from build123d import *

# Parameters (mm, degrees)
F1_DEPTH = 25.4
F2_W     = 101.6
F2_H     = 25.4
F3_DEPTH = 50.8
F4_W     = 25.4
F4_H     = 25.4
F5_DEPTH = 25.401


with BuildPart() as f1:
    # F0 (on Top) → F1 (new body)
    with BuildSketch(Plane.XY):
        with BuildLine():
            ThreePointArc((-50.8, -38.1), (0, -88.9), (50.8, -38.1))
            Line((50.8, -38.1), (25.4, -38.1))
            ThreePointArc((25.4, -38.1), (0, -63.5), (-25.4, -38.1))
            Line((-25.4, -38.1), (-50.8, -38.1))
        make_face()
        with BuildLine():
            ThreePointArc((-50.8, -38.1), (0, 12.7), (50.8, -38.1))
            Line((50.8, -38.1), (50.8, 38.1))
            Line((50.8, 38.1), (-50.8, 38.1))
            Line((-50.8, 38.1), (-50.8, -38.1))
        make_face()
        with BuildLine():
            Line((25.4, -38.1), (50.8, -38.1))
            ThreePointArc((50.8, -38.1), (0, 12.7), (-50.8, -38.1))
            Line((-50.8, -38.1), (-25.4, -38.1))
            ThreePointArc((-25.4, -38.1), (0, -12.7), (25.4, -38.1))
        make_face()
    extrude(amount=F1_DEPTH)

    # F2 (on face) → F3 (join)
    with BuildSketch(Plane.XY.offset(25.4)):
        with Locations((0, 25.4)):
            Rectangle(F2_W, F2_H)
    extrude(amount=F3_DEPTH)

    # F4 (on face) → F5 (cut, through all)
    with BuildSketch(Plane.XZ.offset(-12.7)):
        with Locations((-38.1, 63.5)):
            Rectangle(F4_W, F4_H)
    extrude(amount=-F5_DEPTH, mode=Mode.SUBTRACT)


solid = f1.part
CAD build for the part. Positions are in the model's coordinates, mm. A direction names the side the tool comes from. Round coordinates to 2 decimals unless told otherwise and drop trailing zeros. Order: outer loops, then holes, each group sorted by start corner. A loop starts at its lowest first (then second) coordinate and runs counter-clockwise, first axis right, second up. Notation, with made-up numbers: (-39, 48) -> (-13, 48) arc R16 cw to (-13, 61) -> close; hole circle Ø9 at (61, 41.25). An arc over 180 degrees is marked (long way). Write item = value, one per line. Start each with the question number.
(1) Probe line 1 (Y direction, x = 0, z = 19.5); line 2 (Y direction, x = -43, z = 32.5); line 3 (Z direction, x = -5, y = 12.5). List the from-to ranges inside material, lowest first. Write a range as [from, to].
(2) Pull direction X, two halves, no side cores. Call faces 4 (the cylindrical face through (3.307, -12.916, 12.522)), 5 (the flat face through (-1, 12.7, 50)), 6 (the flat face through (50.8, 16, 29)), 7 (the flat face through (-25.4, 25, 63)): released by +X, released by -X, zero draft, split by the parting line, or undercut.
(3) Cut at D-D, the plane z = 62. List the corners of the cut face in (x, y), then the cut area to 3 significant figures.
(4) Cut at A-A, the plane x = 0. List the corners of the cut face in (y, z), then the cut area to 3 significant figures.
(5) Cut at C-C, the plane z = 21. List the corners of the cut face in (x, y).
(6) Cut at B-B, the plane y = -48. List the corners of the cut face in (x, z), then the cut area to 3 significant figures.
(7) Pin check, flat tips, straight feed: P1, Ø6, axis at x = 23.5, y = -65, coming from the +Z side; P2, Ø4, axis at x = 22.5, y = 16, coming from the -Z side; P3, Ø7.5, axis at y = 25, z = 69, coming from the -X side; P4, Ø20.5, axis at x = -37, y = 31.5, coming from the +Z side. Stop position of each tip, or through.
(8) Which spindle directions (+Z, -Z, +X, -X, +Y, -Y) get a long thin tool onto all of the face, cutting with end or side? Do faces 1 (the flat face through (-38, 25, 50.8)), 2 (the flat face through (11, -15, 25.4)), 3 (the cylindrical face through (-1.117, -88.888, 12.522)). Say none if no direction does.
Model answer:
q1.line_1 = [-88.9, -63.5], [-12.7, 38.1]
q1.line_2 = [12.7, 38.1]
q1.line_3 = [0, 25.4]
q2.face_4 = undercut
q2.face_5 = zero draft
q2.face_6 = released by +X
q2.face_7 = released by -X
q3.outline = (-25.4, 12.7) -> (50.8, 12.7) -> (50.8, 38.1) -> (-25.4, 38.1) -> close
q3.area = 1,940 mm2
q4.outline = (-88.9, 0) -> (-63.5, 0) -> (-63.5, 25.4) -> (-88.9, 25.4) -> close; (-12.7, 0) -> (38.1, 0) -> (38.1, 76.2) -> (12.7, 76.2) -> (12.7, 25.4) -> (-12.7, 25.4) -> close
q4.area = 3,230 mm2
q5.outline = (-50.8, -38.1) arc R50.8 ccw to (50.8, -38.1) -> (50.8, 38.1) -> (-50.8, 38.1) -> close; hole circle Ø50.8 at (0, -38.1)
q6.outline = (-49.83, 0) -> (-23.39, 0) -> (-23.39, 25.4) -> (-49.83, 25.4) -> close; (23.39, 0) -> (49.83, 0) -> (49.83, 25.4) -> (23.39, 25.4) -> close
q6.area = 1,340 mm2
q7.P1 = 25.4
q7.P2 = 0
q7.P3 = -25.4
q7.P4 = 50.8
q8.face_1 = +Z, -X, +Y, -Y
q8.face_2 = +Z, +X, -X, -Y
q8.face_3 = +Z, -Z, -Y
